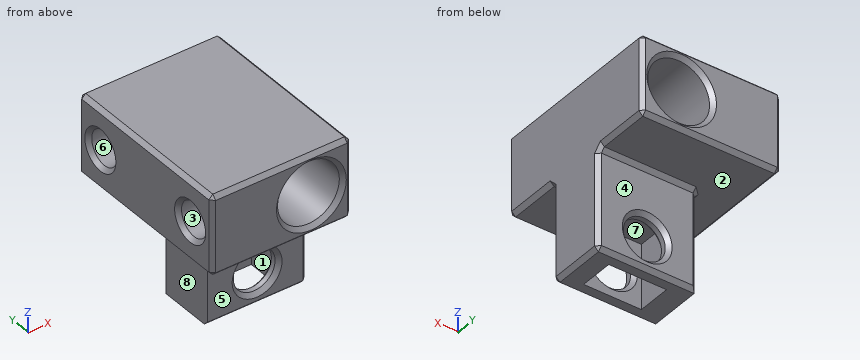
from build123d import *

# Parameters (mm, degrees)
SKETCH1_W               = 35
SKETCH1_H               = 20
BOSS_EXTRUDE1_DEPTH     = 45
SKETCH2_R               = 7.75
CUT_EXTRUDE1_DEPTH      = 46
SKETCH10_R              = 4.25
CUT_EXTRUDE6_DEPTH      = 10
SKETCH4_W               = 25
SKETCH4_H               = 15
BOSS_EXTRUDE2_DEPTH     = 25
SKETCH5_W               = 14.5
SKETCH5_H               = 16.25
CUT_EXTRUDE3_DEPTH      = 31
BOSS_EXTRUDE3_REACH     = 21.75
SKETCH6_W               = 16.25
SKETCH6_H               = 3.25
SKETCH7_R               = 5.25
CUT_EXTRUDE4_DEPTH      = 27.75
CUT_EXTRUDE4_DEPTH_BACK = 19.25
CHAMFER1_SIZE           = 1


with BuildPart() as part:
    # Sketch1 → Boss-Extrude1 (new body)
    with BuildSketch(Plane(origin=(0, 0, 0), x_dir=(1, 0, 0), z_dir=(0, 1, 0))):
        with Locations((17.5, 10)):
            Rectangle(SKETCH1_W, SKETCH1_H)
    extrude(amount=BOSS_EXTRUDE1_DEPTH)

    # Sketch2 → Cut-Extrude1 (cut, through all)
    with BuildSketch(Plane(origin=(0, 45, 0), x_dir=(1, 0, 0), z_dir=(0, 1, 0))):
        with Locations((25, 10)):
            Circle(SKETCH2_R)
    extrude(amount=-CUT_EXTRUDE1_DEPTH, mode=Mode.SUBTRACT)

    # Sketch10 → Cut-Extrude6 (cut)
    with BuildSketch(Plane.ZY):
        with Locations((-10, 37.6875)):
            Circle(SKETCH10_R)
        with Locations((-10, 7.3125)):
            Circle(SKETCH10_R)
    extrude(amount=-CUT_EXTRUDE6_DEPTH, mode=Mode.SUBTRACT)

    # Sketch4 → Boss-Extrude2 (add)
    with BuildSketch(Plane(origin=(0, 0, -20), x_dir=(-1, 0, 0), z_dir=(0, 0, -1))):
        with Locations((-22.5, 22.5)):
            Rectangle(SKETCH4_W, SKETCH4_H)
    extrude(amount=BOSS_EXTRUDE2_DEPTH)

    # Sketch5 → Cut-Extrude3 (cut, through all)
    with BuildSketch(Plane(origin=(0, 30, 0), x_dir=(1, 0, 0), z_dir=(0, 1, 0))):
        with Locations((22.5, 36.875)):
            Rectangle(SKETCH5_W, SKETCH5_H)
    extrude(amount=-CUT_EXTRUDE3_DEPTH, mode=Mode.SUBTRACT)

    # Sketch6 → Boss-Extrude3 (add, up to next)
    with BuildSketch(Plane(origin=(15.25, 0, 0), x_dir=(0, 0, -1), z_dir=(1, 0, 0)), mode=Mode.PRIVATE) as boss_extrude3_sk1:
        with Locations((36.875, 28.375)):
            Rectangle(SKETCH6_W, SKETCH6_H)
    boss_extrude3_tool1 = extrude(boss_extrude3_sk1.sketch, amount=BOSS_EXTRUDE3_REACH, mode=Mode.PRIVATE) - part.part
    add(boss_extrude3_tool1.solids().sort_by_distance((15.25, 28.375, -36.875))[0])
    # Sketch6 → Boss-Extrude3 (add, up to next)
    with BuildSketch(Plane(origin=(15.25, 0, 0), x_dir=(0, 0, -1), z_dir=(1, 0, 0)), mode=Mode.PRIVATE) as boss_extrude3_sk2:
        with Locations((36.875, 16.625)):
            Rectangle(SKETCH6_W, SKETCH6_H)
    boss_extrude3_tool2 = extrude(boss_extrude3_sk2.sketch, amount=BOSS_EXTRUDE3_REACH, mode=Mode.PRIVATE) - part.part
    add(boss_extrude3_tool2.solids().sort_by_distance((15.25, 16.625, -36.875))[0])

    # Sketch7 → Cut-Extrude4 (cut, two sides)
    with BuildSketch(Plane(origin=(0, 18.25, 0), x_dir=(1, 0, 0), z_dir=(0, 1, 0))) as cut_extrude4_sk:
        with Locations((22.5, 36.875)):
            Circle(SKETCH7_R)
    extrude(amount=CUT_EXTRUDE4_DEPTH, mode=Mode.SUBTRACT)
    extrude(cut_extrude4_sk.sketch, amount=-CUT_EXTRUDE4_DEPTH_BACK, mode=Mode.SUBTRACT)

    # Chamfer1
    chamfer1_edges = [part.edges().sort_by_distance(p)[0] for p in [
        (35, 45, -10),
        (17.25, 0, -10),
        (17.25, 45, -10),
        (17.5, 45, -20),
        (0, 37.6875, -14.25),
        (0, 7.3125, -14.25),
        (35, 7.5, -20),
        (10, 22.5, -20),
        (22.5, 30, -20),
        (10, 30, -32.5),
        (35, 30, -32.5),
        (22.5, 15, -20),
        (35, 15, -32.5),
        (22.5, 30, -45),
        (35, 22.5, -45),
        (22.5, 15, -45),
        (0, 45, -10),
        (17.5, 0, -20),
        (35, 0, -10),
        (17.5, 0, 0),
        (0, 0, -10),
        (0, 22.5, -20),
        (35, 37.5, -20),
        (35, 22.5, 0),
        (0, 22.5, 0),
        (17.25, 26.75, -36.875),
        (17.25, 30, -36.875),
        (17.25, 18.25, -36.875),
        (17.25, 15, -36.875),
        (17.5, 45, 0),
    ]]
    chamfer(chamfer1_edges, length=CHAMFER1_SIZE)


solid = part.part
Source: CAD feature listing. Evaluate the final solid. Frame: model axes, mm. Face numbers are marked on the shaded views. A direction names the side the tool comes from. Coordinates: 2 decimals unless noted, no trailing zeros. Order: outer loops, then holes, each group sorted by start corner. A loop starts at its lowest first (then second) coordinate and runs counter-clockwise, first axis right, second up. Notation, with made-up numbers: M 37.5,88 L 95.5,88 A25 cw 95.5,114 Z; hole C 28,18 d1. An arc over 180 degrees is marked long. Write each question's results on one line, items separated by ' | '. Start each with the question number.
Item 1: Cut plane C-C (y = 19). Return loops of the section in (x, z).
Item 2: First-contact query: pin 1 Ø7 at (x, z) = (25.5, -38) entering from +Y; pin 2 Ø4 at (y, z) = (23.5, -36.5) entering from -X; pin 3 Ø16 at (x, z) = (25.5, -33) entering from -Y. Flat tips, straight axial feed; report the tip coordinate or a pass-through.
Item 3: Cut plane B-B (z = -10). Return loops of the section in (x, y), and give its area (4 significant figures).
Item 4: Draft query along Z for the marked faces 1, 2 and 3. Return one class per face: pulls with the +Z half, pulls with the -Z half, needs draft (parallel to the pull), parting line crosses it, or undercut.
Item 5: Set-up query: the marked faces 4, 5, 6, 7 and 8. Return all of +Z, -Z, +X, -X, +Y, -Y with unobstructed straight access to the full face (end or side cutting, diameter ignored); none if empty.
Item 6: Cut plane A-A (z = -29.5). Return loops of the section in (x, y), and give its area (3 significant figures).
Item 7: Cut plane D-D (x = 22.5). Count the separate pieces of the cut face and the enclosed holes in it, and give its area (3 significant figures).
Item 8: Line query: probe 1 along Z at (x, y) = (22.5, 28.3) (3 decimals); probe 2 along Z at (x, y) = (20.5, 15.5); probe 3 along X at (y, z) = (13.5, -10). Output: solid intervals per line, ascending.
Checked values:
1) outline: M 0,-19 L 1,-20 L 9,-20 L 10,-21 L 10,-45 L 15.25,-45 L 15.25,-28.75 L 29.75,-28.75 L 29.75,-45 L 34,-45 L 35,-44 L 35,-1 L 34,0 L 1,0 L 0,-1 Z; hole C 25,-10 d15.5
2) pin 1: stops at y = 30 | pin 2: stops at x = 10 | pin 3: stops at y = 15
3) outline: M 0,1 L 1,0 L 16.25,0 L 17.25,1 L 17.25,44 L 16.25,45 L 1,45 L 0,44 L 0,42.94 L 1,41.94 L 10,41.94 L 10,33.44 L 1,33.44 L 0,32.44 L 0,12.56 L 1,11.56 L 10,11.56 L 10,3.06 L 1,3.06 L 0,2.06 Z; M 32.75,1 L 33.75,0 L 34,0 L 35,1 L 35,44 L 34,45 L 33.75,45 L 32.75,44 Z | area: 701.5 mm2
4) face 1: needs draft | face 2: pulls with the -Z half | face 3: undercut
5) face 4: -Z, +X, -X, +Y | face 5: -Z, +X, -X, -Y | face 6: -X | face 7: -Z | face 8: -Z, -X, +Y, -Y
6) outline: M 10,15 L 34,15 L 35,16 L 35,29 L 34,30 L 11,30 L 10,29 Z; hole M 15.25,18.25 L 29.75,18.25 L 29.75,26.75 L 15.25,26.75 Z | area: 250 mm2
7) separate pieces: 4 | enclosed holes: 0 | area: 400 mm2
8) probe 1: z = -45 to -42.125, -31.625 to -17.336, -2.664 to 0 | probe 2: z = -44.5 to -42.27, -31.48 to -16.31, -3.69 to 0 | probe 3: x = 0 to 17.25, 32.75 to 35
